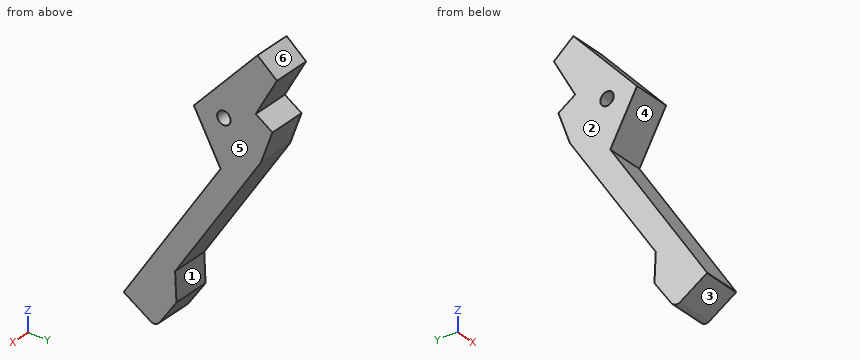
from build123d import *

# Parameters (mm, degrees)
SKETCH_1_R      = 2.1
EXTRUDE_1_DEPTH = 6


with BuildPart() as part:
    # 스케치1 → 보스-돌출1 (new, symmetric)
    with BuildSketch(Plane(origin=(0, 0, 0), x_dir=(0, 0, -1), z_dir=(1, 0, 0))):
        with BuildLine():
            Line((-1.247311697, 15.290072814), (-4.747158569, 10.027630369))
            Line((-4.747158569, 10.027630369), (-16.737908316, 16.712025722))
            Line((-16.737908316, 16.712025722), (-21.94836762, 10.590510846))
            Line((-21.94836762, 10.590510846), (-0.281769869, -9.435112952))
            Line((-0.281769869, -9.435112952), (15.1257089, -1.028923277))
            Line((15.1257089, -1.028923277), (61.632849993, -31.445174091))
            Line((61.632849993, -31.445174091), (61.80599614, -31.445174091))
            Line((61.80599614, -31.445174091), (67.317930071, -22.846306867))
            ThreePointArc((67.317930071, -22.846306867), (67.40457501, -21.419938181), (66.570574662, -20.259559625))
            Line((66.570574662, -20.259559625), (58.8607522, -14.920439997))
            Line((58.8607522, -14.920439997), (49.925171415, -15.334910855))
            Line((49.925171415, -15.334910855), (8.746820412, 11.671154757))
            Line((8.746820412, 11.671154757), (-1.247311697, 15.290072814))
        make_face()
        Circle(SKETCH_1_R, mode=Mode.SUBTRACT)
    extrude(amount=EXTRUDE_1_DEPTH, both=True)


solid = part.part
Source: CAD feature listing. Evaluate the final solid. Frame: model axes, mm. Face numbers are marked on the shaded views. A direction names the side the tool comes from. Coordinates: 2 decimals unless noted, no trailing zeros. Order: outer loops, then holes, each group sorted by start corner. A loop starts at its lowest first (then second) coordinate and runs counter-clockwise, first axis right, second up.
Item 1: Cut plane B-B (y = 0). Return loops of the section in (x, z).
Output values:
outline: (-6, -26.54) - (6, -26.54) - (6, -2.1) - (-6, -2.1) - close; (-6, 2.1) - (6, 2.1) - (6, 10.49) - (-6, 10.49) - close
Item 2: Pull-direction query (Z, two-part tool) for the marked faces 3, 4, 5 and 6; classes: pulls with the +Z half, pulls with the -Z half, needs draft (parallel to the pull), parting line crosses it, or undercut.
Output values:
face 3: pulls with the -Z half
face 4: undercut
face 5: needs draft
face 6: pulls with the +Z half
Item 3: Cut plane C-C (z = 9). Return loops of the section in (x, y), plus the area to 3 significant figures.
Output values:
outline: (-6, -1.38) - (6, -1.38) - (6, 12.4) - (-6, 12.4) - close
area: 165 mm2
Item 4: Cut plane D-D (y = -18). Return loops of the section in (x, z), plus the area to 3 significant figures.
Output values:
outline: (-6, -63.31) - (6, -63.31) - (6, -41.07) - (-6, -41.07) - close
area: 267 mm2
Item 5: Set-up query: the marked faces 1 and 2. Return all of +Z, -Z, +X, -X, +Y, -Y with unobstructed straight access to the full face (end or side cutting, diameter ignored); none if empty.
Output values:
face 1: +X, -X, +Y
face 2: +Z, -Z, -X, +Y, -Y
Item 6: Material intervals for line 1 (Y direction, x = 2.75, z = 0); line 2 (Z direction, x = 5.75, y = -6.5); line 3 (Y direction, x = 2.75, z = -29), sorted ascending.
Output values:
line 1: y = -9.28 to -2.1, 2.1 to 14.84
line 2: z = -36.45 to -23.49, -5.1 to 3.46
line 3: y = -10.1 to -1.61
Item 7: First-contact query: P1, Ø3, axis at x = -3.5, y = -10.5, coming from the +Z side; P2, Ø6, axis at x = -3, z = -23.5, coming from the +Y side; P3, Ø3, axis at x = -2.5, z = -40.5, coming from the -Y side; P4, Ø4, axis at y = -18.5, z = -40.5, coming from the +X side. Flat tips, straight axial feed; report the tip coordinate or a pass-through.
Output values:
P1: stops at z = 0.75
P2: stops at y = 3.96
P3: stops at y = -18.61
P4: stops at x = 6
Item 8: Cut plane A-A (x = -3.25). Return loops of the section in (y, z).
Output values:
outline: (-31.45, -61.81) - (-22.85, -67.32) arc R2.13 ccw to (-20.26, -66.57) - (-14.92, -58.86) - (-15.33, -49.93) - (11.67, -8.75) - (15.29, 1.25) - (10.03, 4.75) - (16.71, 16.74) - (10.59, 21.95) - (-9.44, 0.28) - (-1.03, -15.13) - (-31.45, -61.63) - close; hole circle Ø4.2 at (0, 0)
